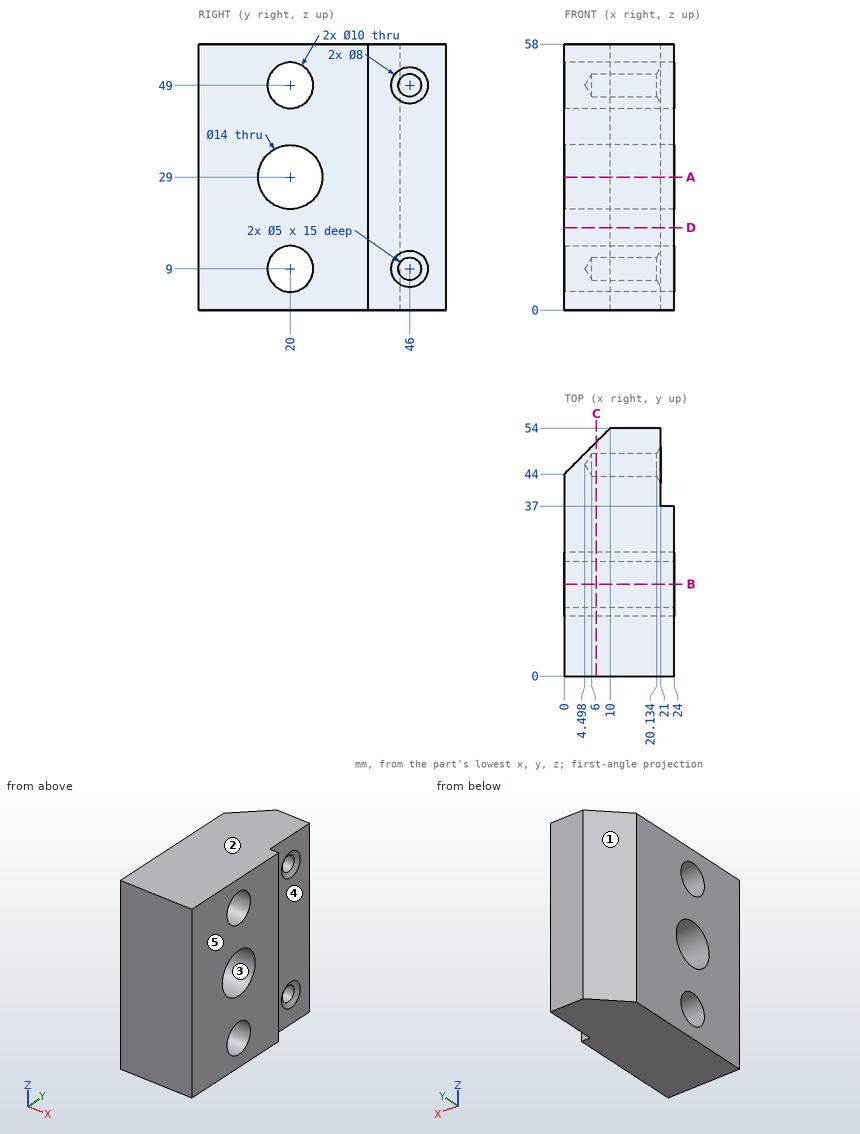
Study the drawing (mm; zero at the part's minimum x, y, z) and answer. A direction names the side the tool comes from. Coordinates: 2 decimals unless noted, no trailing zeros. Order: outer loops, then holes, each group sorted by start corner. A loop starts at its lowest first (then second) coordinate and runs counter-clockwise, first axis right, second up. Notation, with made-up numbers: M 22.5,54 L 48.5,54 A18 ccw 48.5,73 Z; hole C 37.25,72.5 d2. An arc over 180 degrees is marked long. Answer as a JSON object with one key per item and string values. Group by question number.
1. Straight lines are drawn through the part: line 1 (Y direction, x = 12, z = 9); line 2 (Y direction, x = 15.5, z = 29); line 3 (Y direction, x = 19.75, z = 10). For each, find the intervals that lie inside material, in ascending order.
2. Section B-B on y = 20 is taken. Write down the section's boundary in (x, z), then the cut area to 3 significant figures.
3. Determine the mould class of the marked faces 1, 2 and 3 for opening direction Y: released by +Y, released by -Y, zero draft, split by the parting line, or undercut.
4. Section D-D on z = 18 is taken. Write down the section's boundary in (x, y).
5. Section A-A on z = 29 is taken. Write down the section's boundary in (x, y), then the cut area to 3 significant figures.
6. Section C-C on x = 7 is taken. Write down the section's boundary in (y, z), then the cut area to 3 significant figures.
7. A tool of negligible diameter and unlimited length cuts with its end or side. For the marked faces 4 and 5, from which of +Z, -Z, +X, -X, +Y, -Y can it reach the whole face along a straight path? Write none if from no direction.
8. Flat-ended cylindrical pins translate along their axes: P1, Ø0.9, axis at x = 22, z = 32, coming from the +Y side; P2, Ø6, axis at y = 46, z = 49, coming from the +X side; P3, Ø8, axis at y = 44, z = 50.5, coming from the +X side. Find the tip coordinate at first contact, or state that the pin passes through.
Values follow:
{
 "1": {"line 1": "0 to 15, 25 to 43.5, 48.5 to 54", "line 2": "0 to 13, 27 to 54", "line 3": "0 to 15.1, 24.9 to 43.71, 48.29 to 54"},
 "2": {"outline": "M 0,0 L 24,0 L 24,4 L 0,4 Z; M 0,14 L 24,14 L 24,22 L 0,22 Z; M 0,36 L 24,36 L 24,44 L 0,44 Z; M 0,54 L 24,54 L 24,58 L 0,58 Z", "area": "576 mm2"},
 "3": {"face 1": "released by +Y", "face 2": "zero draft", "face 3": "undercut"},
 "4": {"outline": "M 0,0 L 24,0 L 24,37 L 21,37 L 21,54 L 10,54 L 0,44 Z"},
 "5": {"outline": "M 0,0 L 24,0 L 24,13 L 0,13 Z; M 0,27 L 24,27 L 24,37 L 21,37 L 21,54 L 10,54 L 0,44 Z", "area": "859 mm2"},
 "6": {"outline": "M 0,0 L 51,0 L 51,58 L 0,58 Z; hole C 20,29 d14; hole C 20,9 d10; hole C 20,49 d10; hole C 46,9 d5; hole C 46,49 d5", "area": "2,610 mm2"},
 "7": {"face 4": "+Z, -Z, +X, +Y", "face 5": "+Z, -Z, +X, +Y, -Y"},
 "8": {"P1": "y = 37", "P2": "x = 20.42", "P3": "x = 21"}
}
